Design review of the part built by this model. Coordinates are the model's own, in mm. A direction names the side the tool comes from. Round coordinates to 2 decimals unless told otherwise and drop trailing zeros. Loops run counter-clockwise (first coordinate to the right, second up) from the corner with the lowest first, then second, coordinate; pieces in that order, holes last. Notation, with made-up numbers: (-23, 59) - (-14, 59) arc R10 cw to (-14, 77) - close; hole circle Ø4 at (-27.75, -34.5). An arc over 180 degrees is marked (long way). Return JSON: item names as keys, results as strings. Group by question number.
(1) For faces 4 (the flat face through (-8.5, -15.5, 40)), 5 (the flat face through (9, 10, 33)), 6 (the flat face through (0, -43, 20)), 7 (the flat face through (28.3, 30, 0)), 8 (the flat face through (43, -5, 10)), list the 3-axis set-ups (+Z, -Z, +X, -X, +Y, -Y) from which the entire face can be reached by the end or side of a thin tool; tool diameter is ignored.
(2) We need section B-B, the plane x = 0. Write out the cut boundary in (y, z), and give its area (3 significant figures).
(3) The part is to be moulded in two halves that separate along Y. For faces 1 (the flat face through (5, 43, 10)), 2 (the cylindrical face through (-13.887, 10.648, 49.86)), 3 (the flat face through (-43, 5, 10)), say which applies: pulls with the +Y half, pulls with the -Y half, needs draft (parallel to the pull), parting line crosses it, or undercut.
(4) Clearance check with flat-ended pins moving along their axes: pin 1 (4 mm diameter, centred on y = -44, z = 12.5, fed in from -X); pin 2 (8 mm diameter, centred on y = 32, z = 7.5, fed in from +X); pin 3 (10 mm diameter, centred on x = -31, z = 7.5, fed in from +Y); pin 4 (1.5 mm diameter, centred on x = 28.5, y = -33.5, fed in from -Z). State where each tip first meets the part, or that it passes through.
(5) Wall thickness on L1, parallel to Y at x = 0, z = 51; L2, parallel to X at y = 22, z = 14; L3, parallel to Z at x = 11, y = -6.5: over which ranges is each line inside the solid? List them lowest first. Write a range as [from, to].
(6) We need section D-D, the plane z = 56.5. Write out the cut boundary in (x, y).
(7) We need section A-A, the plane z = 16. Write out the cut boundary in (x, y), and give its area (3 significant figures).
Autodesk Inventor part; units mm, degrees
ref_plane "Work Plane1" through (0, -46, 0) normal (0, 1, 0) x (-1, 0, 0)
ref_plane "Work Plane2" through (46, 0, 0) normal (1, 0, 0) x (0, 1, 0)
ref_plane "XY Plane" through (0, 0, 0) normal (0, 0, 1) x (1, 0, 0)
sketch "Sketch1" plane through (0, 0, 0) normal (0, 0, 1) x (1, 0, 0)
  circle A0 centre (0, 0) radius 41
  circle A1 centre (0, 0) radius 12.5
  circle A2 centre (0, 0) radius 46
  dimension "d0" = 82
  dimension "d1" = 25
  dimension "d2" = 92
extrude "Extrusion1" add sketch "Sketch1" along normal blind 40 contours A0 | A2
fillet "Fillet1" radius 10 1 edges at (-46, 0, 40)
extrude "Extrusion2" cut sketch "Sketch1" along normal blind 33 contours A0
sketch "Sketch2" plane through (0, 0, 40) normal (0, 0, 1) x (1, 0, 0)
  circle A0 centre (0, 0) radius 17.5
  dimension "d8" = 35
extrude "Extrusion3" add sketch "Sketch2" along normal blind 20
extrude "Extrusion4" cut sketch "Sketch1" along normal blind 118.5 contours A1
thread "Thread1"
ref_plane "Work Plane1" through (0, -46, 0) normal (0, 1, 0) x (-1, 0, 0)
ref_plane "Work Plane2" through (46, 0, 0) normal (1, 0, 0) x (0, 1, 0)
sketch "Sketch3" plane through (0, -46, 0) normal (0, 1, 0) x (-1, 0, 0)
  line L0 (5, 20) -> (-5, 20)
  line L1 (-5, 20) -> (-5, -20)
  line L2 (-5, -20) -> (5, -20)
  line L3 (5, -20) -> (5, 20)
  line L4 (5, 20) -> (-5, -20) construction
  line L5 (-5, 20) -> (5, -20) construction
  point P0 (0, 0)
  dimension "d15" = 10
  dimension "d16" = 40
extrude "Extrusion5" cut sketch "Sketch3" along normal blind 154.5
sketch "Sketch4" plane through (46, 0, 0) normal (1, 0, 0) x (0, 1, 0)
  line L0 (-5, 20) -> (5, 20)
  line L1 (5, 20) -> (5, -20)
  line L2 (5, -20) -> (-5, -20)
  line L3 (-5, -20) -> (-5, 20)
  line L4 (-5, 20) -> (5, -20) construction
  line L5 (5, 20) -> (-5, -20) construction
  point P0 (0, 0)
  dimension "d19" = 10
  dimension "d20" = 40
extrude "Extrusion6" cut sketch "Sketch4" against normal blind 154.5
properties part number "input"
Solutions:
{
 "1": {"face 4": "+Z", "face 5": "-Z", "face 6": "-Z, +Y, -Y", "face 7": "-Z, +X, -X, +Y, -Y", "face 8": "-Z, +X, -X"},
 "2": {"outline": "(-46, 20) - (-41, 20) - (-41, 33) - (-12.5, 33) - (-12.5, 60) - (-17.5, 60) - (-17.5, 40) - (-36, 40) arc R10 ccw to (-46, 30) - close; (12.5, 33) - (41, 33) - (41, 20) - (46, 20) - (46, 30) arc R10 ccw to (36, 40) - (17.5, 40) - (17.5, 60) - (12.5, 60) - close", "area": "756 mm^2"},
 "3": {"face 1": "needs draft", "face 2": "parting line crosses it", "face 3": "undercut"},
 "4": {"pin 1": "x = -18.76", "pin 2": "x = 36.5", "pin 3": "y = 37.95", "pin 4": "z = 0"},
 "5": {"L1": "[-17.5, -12.5], [12.5, 17.5]", "L2": "[-40.4, -34.6], [34.6, 40.4]", "L3": "[33, 60]"},
 "6": {"outline": "circle Ø35 at (0, 0); hole circle Ø25 at (0, 0)"},
 "7": {"outline": "(-45.73, -5) arc R46 ccw to (-5, -45.73) - (-5, -40.69) arc R41 cw to (-40.69, -5) - close; (-45.73, 5) - (-40.69, 5) arc R41 cw to (-5, 40.69) - (-5, 45.73) arc R46 ccw to start; (5, -45.73) arc R46 ccw to (45.73, -5) - (40.69, -5) arc R41 cw to (5, -40.69) - close; (5, 40.69) arc R41 cw to (40.69, 5) - (45.73, 5) arc R46 ccw to (5, 45.73) - close", "area": "1,170 mm^2"}
}
